Read the model definition and answer for the solid it produces. Units are mm, in the model's axes. A direction names the side the tool comes from. Coordinates: 2 decimals unless noted, no trailing zeros. Loops run counter-clockwise (first coordinate to the right, second up) from the corner with the lowest first, then second, coordinate; pieces in that order, holes last. Notation, with made-up numbers: (-21, 14.5) - (38, 14.5) arc R11 cw to (38, 30.5) - close; hole circle Ø4 at (68, 72). An arc over 180 degrees is marked (long way). Use one line per item in the form item = value.
from build123d import *

# Parameters (mm, degrees)
F0_W          = 25.4
F0_H          = 3.175
F1_DEPTH      = 19.05
F3_DEPTH      = 25.4
F3_DEPTH_BACK = 19.05
F4_W          = 25.4
F4_H          = 9.525
F5_DEPTH      = 2.54
F6_W          = 19.05
F6_H          = 1.5875
F7_DEPTH      = 6.35


with BuildPart() as f1:
    # F0 (on Top) → F1 (new body)
    with BuildSketch(Plane.XY):
        with Locations((12.7, 1.5875)):
            Rectangle(F0_W, F0_H)
    extrude(amount=F1_DEPTH)

    # F2 (on face) → F3 (join, two sides)
    with BuildSketch(Plane(origin=(0, 0, 0), x_dir=(1, 0, 0), z_dir=(0, 0, -1))) as f3_sk:
        Polygon((25.4, -9.525), (25.4, -3.175), (0, -3.175), (0, -9.525), (1.5875, -9.525), (3.175, -9.525), (3.175, -7.9375), (1.5875, -7.9375), (1.5875, -4.7625), (23.8125, -4.7625), (23.8125, -7.9375), (22.225, -7.9375), (22.225, -9.525), (23.8125, -9.525), align=None)
    extrude(amount=F3_DEPTH)
    extrude(f3_sk.sketch, amount=-F3_DEPTH_BACK)

    # F4 (on face) → F5 (join)
    with BuildSketch(Plane.XY.offset(19.05)):
        with Locations((12.7, 4.7625)):
            Rectangle(F4_W, F4_H)
    extrude(amount=-F5_DEPTH)

    # F6 (on face) → F7 (cut)
    with BuildSketch(Plane(origin=(0, 0, -25.4), x_dir=(1, 0, 0), z_dir=(0, 0, -1))):
        with Locations((12.7, -3.96875)):
            Rectangle(F6_W, F6_H)
    extrude(amount=-F7_DEPTH, mode=Mode.SUBTRACT)


solid = f1.part
Item 1: The part is cut by section B-B on y = 6. Give the vertices of the cut face in (x, z).
Results below:
outline = (0, -25.4) - (1.59, -25.4) - (1.59, 16.51) - (23.81, 16.51) - (23.81, -25.4) - (25.4, -25.4) - (25.4, 19.05) - (0, 19.05) - close
Item 2: The part is cut by section D-D on z = 4. Give the vertices of the cut face in (x, y) (1 decimal), plus the area to 3 significant figures.
Results below:
outline = (0, 0) - (25.4, 0) - (25.4, 9.5) - (22.2, 9.5) - (22.2, 7.9) - (23.8, 7.9) - (23.8, 4.8) - (1.6, 4.8) - (1.6, 7.9) - (3.2, 7.9) - (3.2, 9.5) - (0, 9.5) - close
area = 141 mm²
Item 3: The part is cut by section A-A on z = -1. Give the vertices of the cut face in (x, y) (1 decimal), plus the area to 3 significant figures.
Results below:
outline = (0, 3.2) - (25.4, 3.2) - (25.4, 9.5) - (22.2, 9.5) - (22.2, 7.9) - (23.8, 7.9) - (23.8, 4.8) - (1.6, 4.8) - (1.6, 7.9) - (3.2, 7.9) - (3.2, 9.5) - (0, 9.5) - close
area = 60.5 mm²
Item 4: Find the intervals of material crossed by L1, parallel to X at y = 5.25, z = -24; L2, parallel to X at y = 8.5, z = 2 (3 decimals); L3, parallel to Z at x = 14.25, y = 8, in increasing order.
Results below:
L1 = 0 to 1.59, 23.81 to 25.4
L2 = 0 to 3.175, 22.225 to 25.4
L3 = 16.51 to 19.05
Item 5: For a pull along Y with two mould halves and no side action, classify faces 6 (the flat face through (23.812, 6, -5)), 7 (the flat face through (13, 3.175, -10)), 8 (the flat face through (1, 6, -25.4)) as +Y half, -Y half, draft (parallel to the pull), parting line (faces both ways), or undercut.
Results below:
face_6 = undercut
face_7 = -Y half
face_8 = draft
Item 6: Each of these flat-tipped pins is pushed along its axis until it touches: P1, Ø12.5, axis at x = 13, z = -15, coming from the -Y side (3 decimals); P2, Ø5, axis at x = 12.5, y = 2, coming from the -Z side; P3, Ø3, axis at x = 13, z = 8.5, coming from the +Y side. Where does it stop, or does it pass through?
Results below:
P1 = 3.175
P2 = -19.05
P3 = 4.76
Item 7: Which of the six approach directions +Z, -Z, +X, -X, +Y, -Y give full straight-line access (tool end or side, diameter ignored) to faces 1 (the flat face through (22.225, 4, -22)), 2 (the flat face through (13, 2, 0)), 3 (the flat face through (3.175, 9, -5)), 4 (the flat face through (13, 4.762, -5)), 5 (the flat face through (25.4, 6, -3))?
Results below:
face_1 = -Z, +Y, -Y
face_2 = -Z, +X, -X, -Y
face_3 = -Z, +Y
face_4 = -Z
face_5 = +Z, -Z, +X, +Y, -Y
